Could you check a few things on this model? Use its own coordinates, in mm. A direction names the side the tool comes from. Give positions to 0.01 mm unless a question says otherwise; leave off trailing zeros. Order: outer loops, then holes, each group sorted by start corner. A loop starts at its lowest first (then second) coordinate and runs counter-clockwise, first axis right, second up.
from build123d import *

# Parameters (mm, degrees)
F0_W     = 23
F0_H     = 36.5
F1_DEPTH = 1.58
F2_W     = 8
F2_H     = 5
F3_DEPTH = 3
F2_W_2   = 6
F2_H_2   = 8
F4_DEPTH = 5
F5_R     = 1.5


with BuildPart() as f1:
    # F0 (on Top) → F1 (new body)
    with BuildSketch(Plane.XY):
        Rectangle(F0_W, F0_H)
    extrude(amount=F1_DEPTH)

    # F2 (on face) → F3 (join)
    with BuildSketch(Plane.XY.offset(1.58)):
        with Locations((0, -15.75)):
            Rectangle(F2_W, F2_H)
    extrude(amount=F3_DEPTH)

    # F2 (on face) → F4 (join)
    with BuildSketch(Plane.XY.offset(1.58)):
        with Locations((-8.5, -6.85)):
            Rectangle(F2_W_2, F2_H_2)
    extrude(amount=F4_DEPTH)

    # F5
    f5_edges = [f1.edges().sort_by_distance(p)[0] for p in [
        (-11.5, -18.25, 0.79),
        (11.5, -18.25, 0.79),
        (11.5, 18.25, 0.79),
        (-11.5, 18.25, 0.79),
    ]]
    fillet(f5_edges, radius=F5_R)


solid = f1.part
Item 1: Imagine slicing it at B-B on y = -14. List the corners of the cut face in (x, z) for me.
Findings:
outline: (-11.5, 0) - (11.5, 0) - (11.5, 1.58) - (4, 1.58) - (4, 4.58) - (-4, 4.58) - (-4, 1.58) - (-11.5, 1.58) - close
Item 2: Please list where these lines run through material, in increasing order: line 1 along Z through (x, y) = (7.5, -13); line 2 along X through (y, z) = (-10.5, 4.75); line 3 along Y through (x, z) = (-3.5, 3.5).
Findings:
line 1: z = 0 to 1.58
line 2: x = -11.5 to -5.5
line 3: y = -18.25 to -13.25
Item 3: Imagine slicing it at A-A on z = 3.75. List the corners of the cut face in (x, y) for me, then the cut area to 3 significant figures.
Findings:
outline: (-11.5, -10.85) - (-5.5, -10.85) - (-5.5, -2.85) - (-11.5, -2.85) - close; (-4, -18.25) - (4, -18.25) - (4, -13.25) - (-4, -13.25) - close
area: 88.0 mm2
Item 4: For pin 1 (0.9 mm diameter, centred on x = 0, z = 3.5, fed in from +Y); pin 2 (5 mm diameter, centred on x = 5, y = -10, fed in from +Z); pin 3 (2.5 mm diameter, centred on x = -7.5, z = 4, fed in from -Y), each with a flat end and sliding along its axis, tell me the tip position at first contact or that it passes through.
Findings:
pin 1: stops at y = -13.25
pin 2: stops at z = 1.58
pin 3: stops at y = -10.85
Item 5: For faces 1 (the flat face through (-9, -10.85, 4)), 2 (the flat face through (-4, -16, 3)), 3 (the cylindrical face through (11.05, -17.82, 0.8)), 4 (the flat face through (-9, -2.85, 4)), 5 (the flat face through (4, -16, 3)), which set-ups out of +Z, -Z, +X, -X, +Y, -Y let a thin tool reach every point of the face, with its end or its side?
Findings:
face 1: +Z, +X, -X, -Y
face 2: +Z, -X, +Y, -Y
face 3: +Z, -Z, +X, -Y
face 4: +Z, +X, -X, +Y
face 5: +Z, +X, +Y, -Y
Item 6: Imagine slicing it at C-C on x = 1.5. List the corners of the cut face in (y, z) for me, then the cut area to 3 significant figures.
Findings:
outline: (-18.25, 0) - (18.25, 0) - (18.25, 1.58) - (-13.25, 1.58) - (-13.25, 4.58) - (-18.25, 4.58) - close
area: 72.7 mm2
Item 7: Imagine slicing it at D-D on x = -8.75. List the corners of the cut face in (y, z) for me.
Findings:
outline: (-18.25, 0) - (18.25, 0) - (18.25, 1.58) - (-2.85, 1.58) - (-2.85, 6.58) - (-10.85, 6.58) - (-10.85, 1.58) - (-18.25, 1.58) - close
